CAD build for the part. Positions are in the model's coordinates, mm. A direction names the side the tool comes from. Round coordinates to 2 decimals unless told otherwise and drop trailing zeros. Write each loop counter-clockwise with the first axis right and the second up, starting at its lowest first coordinate (ties: lowest second). Pieces come first, ordered by that corner, then holes. Notation, with made-up numbers: (13.5, -17.5) - (67.5, -17.5) arc R18 ccw to (67.5, 1.5) - close; hole circle Ø2 at (67.25, -36). An arc over 180 degrees is marked (long way). Put each result on its own line as item: value. Start each with the question number.
Item 1: 3-axis set-ups, long thin cutter, end or side, ignore diameter. For faces 4 (the cylindrical face through (-20.8, -28.1, 0.8)), 5 (the flat face through (25, -1, 1)): which of +Z, -Z, +X, -X, +Y, -Y reach the whole face in a straight line?
Item 2: Drill centre lines: line 1 (Y direction, x = 18.25, z = 1.15); line 2 (X direction, y = -31, z = 0.85); line 3 (Y direction, x = -20, z = 0.75). Where is each one in solid material? Low to high. Write a range as from..to.
Item 3: Cut at A-A (z = 0.5). Give the cut face in (x, y), and give its area (3 significant figures).
Item 4: Mould opens along Y. For faces 1 (the flat face through (-25, 1, 1)), 2 (the cylindrical face through (20.8, -32.9, 0.8)), 3 (the flat face through (0, -37.5, 1)) say: released by +Y, released by -Y, zero draft, split by the parting line, or undercut.
Item 5: Pin check, flat tip, straight feed: pin 1 Ø1.2 at (x, y) = (18.25, 30.5) entering from +Z. Stop position of the tip, or through.
Autodesk Inventor part; units mm, degrees
ref_plane "YZ Plane" through (0, 0, 0) normal (1, 0, 0) x (0, 1, 0)
ref_plane "XZ Plane" through (0, 0, 0) normal (0, 1, 0) x (-1, 0, 0)
ref_plane "XY Plane" through (0, 0, 0) normal (0, 0, 1) x (1, 0, 0)
sketch "Sketch1" plane through (0, 0, 0) normal (0, 0, 1) x (1, 0, 0)
  line L0 (25, 37.5) -> (-25, 37.5)
  line L1 (-25, 37.5) -> (-25, -37.5)
  line L2 (-25, -37.5) -> (25, -37.5)
  line L3 (25, -37.5) -> (25, 37.5)
  line L4 (25, 37.5) -> (-25, -37.5) construction
  line L5 (-25, 37.5) -> (25, -37.5) construction
  line L6 (-20.75, -30.5) -> (20.75, -30.5) construction
  line L7 (20.75, -30.5) -> (20.75, 30.5) construction
  line L8 (20.75, 30.5) -> (-20.75, 30.5) construction
  line L9 (-20.75, 30.5) -> (-20.75, -30.5) construction
  line L10 (-20.75, -30.5) -> (20.75, 30.5) construction
  line L11 (20.75, -30.5) -> (-20.75, 30.5) construction
  circle A0 centre (20.75, 30.5) radius 2.4
  arc A1 (23.0395, 29.7801) -> (23.0395, 31.2199) centre (23.25, 30.5) ccw
  line L12 (0, 37.5) -> (0, -37.5) construction
  line L13 (25, 0) -> (-25, 0) construction
  circle A2 centre (20.75, -30.5) radius 2.4
  arc A3 (23.0395, -31.2199) -> (23.0395, -29.7801) centre (23.25, -30.5) ccw
  line L14 (0, -37.5) -> (0, 37.5) construction
  circle A4 centre (-20.75, 30.5) radius 2.4
  arc A5 (-23.0395, 31.2199) -> (-23.0395, 29.7801) centre (-23.25, 30.5) ccw
  circle A6 centre (-20.75, -30.5) radius 2.4
  arc A7 (-23.0395, -29.7801) -> (-23.0395, -31.2199) centre (-23.25, -30.5) ccw
  arc A8 (18.4605, 31.2199) -> (18.4605, 29.7801) centre (18.25, 30.5) ccw
  arc A9 (18.4605, -29.7801) -> (18.4605, -31.2199) centre (18.25, -30.5) ccw
  arc A10 (-18.4605, 29.7801) -> (-18.4605, 31.2199) centre (-18.25, 30.5) ccw
  arc A11 (-18.4605, -31.2199) -> (-18.4605, -29.7801) centre (-18.25, -30.5) ccw
  point P0 (0, 0)
  point P1 (24, 30.5)
  point P2 (17.5, 30.5)
  point P3 (18.4605, 29.7801)
  point P4 (18.4605, 31.2199)
  point P5 (18.4605, -31.2199)
  point P6 (18.4605, -29.7801)
  point P7 (-18.4605, -29.7801)
  point P8 (-18.4605, -31.2199)
  point P9 (-18.4605, 31.2199)
  point P10 (-18.4605, 29.7801)
  dimension "d0" = 50
  dimension "d1" = 75
  dimension "d2" = 4.8
  dimension "d4" = 1.5
  dimension "d6" = 14
  dimension "d9" = 61
  dimension "d10" = 41.5
  dimension "d11" = 6.5
  dimension "d12" = 1
extrude "Extrusion1" add sketch "Sketch1" along normal blind 1.6
properties part number "SUSTAINA-POWER-INPUT-BORAD" material "CFRP"
Output values:
1. face 4: +Z, -Z
1. face 5: +Z, -Z, +X, +Y, -Y
2. line 1: -37.5..-31.25, -29.75..29.75, 31.25..37.5
2. line 2: -25..-23.81, -17.69..17.69, 23.81..25
2. line 3: -37.5..-32.78, -28.22..28.22, 32.78..37.5
3. outline: (-25, -37.5) - (25, -37.5) - (25, 37.5) - (-25, 37.5) - close; hole (-23.04, -31.22) arc R2.4 ccw to (-18.46, -31.22) arc R0.75 ccw (long way) to (-18.46, -29.78) arc R2.4 ccw to (-23.04, -29.78) arc R0.75 ccw (long way) to start; hole (-23.04, 29.78) arc R2.4 ccw to (-18.46, 29.78) arc R0.75 ccw (long way) to (-18.46, 31.22) arc R2.4 ccw to (-23.04, 31.22) arc R0.75 ccw (long way) to start; hole (18.46, -31.22) arc R2.4 ccw to (23.04, -31.22) arc R0.75 ccw (long way) to (23.04, -29.78) arc R2.4 ccw to (18.46, -29.78) arc R0.75 ccw (long way) to start; hole (18.46, 29.78) arc R2.4 ccw to (23.04, 29.78) arc R0.75 ccw (long way) to (23.04, 31.22) arc R2.4 ccw to (18.46, 31.22) arc R0.75 ccw (long way) to start
3. area: 3,670 mm2
4. face 1: zero draft
4. face 2: undercut
4. face 3: released by -Y
5. pin 1: through
